from build123d import *

# Parameters (mm, degrees)
SKETCH1_R           = 16.5
BOSS_EXTRUDE1_DEPTH = 40
SKETCH2_R           = 1.25
CUT_EXTRUDE1_DEPTH  = 5
SKETCH3_R           = 5
BOSS_EXTRUDE2_DEPTH = 2.5
BOSS_EXTRUDE3_DEPTH = 8.5
CUT_EXTRUDE2_DEPTH  = 2
CUT_EXTRUDE3_START  = -16
SKETCH6_R           = 17.194108904
SKETCH6_R_2         = 15.5
CUT_EXTRUDE3_DEPTH  = 2
FILLET1_R           = 2
SKETCH7_R           = 4.1
BOSS_EXTRUDE4_DEPTH = 3
SKETCH8_R           = 2.5
BOSS_EXTRUDE5_DEPTH = 1
SKETCH9_W           = 3
SKETCH9_H           = 1
BOSS_EXTRUDE6_DEPTH = 6
CUT_EXTRUDE4_DEPTH  = 62.184148274
SKETCH11_W          = 1.5
SKETCH11_H          = 2.5
CUT_EXTRUDE5_DEPTH  = 62.184148274
CUT_EXTRUDE6_DEPTH  = 3.85
FILLET2_R           = 1


with BuildPart() as part:
    # Sketch1 → Boss-Extrude1 (new body)
    with BuildSketch(Plane.XY):
        Circle(SKETCH1_R)
    extrude(amount=BOSS_EXTRUDE1_DEPTH)

    # Sketch2 → Cut-Extrude1 (cut)
    with BuildSketch(Plane.XY.offset(40)):
        with Locations((0, 14)):
            Circle(SKETCH2_R)
        with Locations((12.124355653, -7)):
            Circle(SKETCH2_R)
        with Locations((-12.124355653, -7)):
            Circle(SKETCH2_R)
    extrude(amount=-CUT_EXTRUDE1_DEPTH, mode=Mode.SUBTRACT)

    # Sketch3 → Boss-Extrude2 (add)
    with BuildSketch(Plane.XY.offset(40)):
        with Locations((0, -7)):
            Circle(SKETCH3_R)
    extrude(amount=BOSS_EXTRUDE2_DEPTH)

    # Sketch4 → Boss-Extrude3 (add)
    with BuildSketch(Plane.XY.offset(42.5)):
        with BuildLine():
            Line((-2, -8.5), (2, -8.5))
            ThreePointArc((2, -8.5), (0, -4.5), (-2, -8.5))
        make_face()
    extrude(amount=BOSS_EXTRUDE3_DEPTH)

    # Sketch5 → Cut-Extrude2 (cut)
    with BuildSketch(Plane.XY.offset(40)):
        with BuildLine():
            Line((-13.5, 2.25), (-17.622574656, 2.25))
            Line((-17.622574656, 2.25), (-17.622574656, -2.25))
            Line((-17.622574656, -2.25), (-13.5, -2.25))
            ThreePointArc((-13.5, -2.25), (-11.25, 0), (-13.5, 2.25))
        make_face()
        with BuildLine():
            Line((17.622574656, -2.25), (13.5, -2.25))
            ThreePointArc((13.5, -2.25), (11.25, 0), (13.5, 2.25))
            Line((13.5, 2.25), (17.622574656, 2.25))
            Line((17.622574656, 2.25), (17.622574656, -2.25))
        make_face()
    extrude(amount=-CUT_EXTRUDE2_DEPTH, mode=Mode.SUBTRACT)

    # Sketch6 → Cut-Extrude3 (cut)
    with BuildSketch(Plane.XY.offset(40).offset(CUT_EXTRUDE3_START)):
        Circle(SKETCH6_R)
        Circle(SKETCH6_R_2, mode=Mode.SUBTRACT)
    extrude(amount=-CUT_EXTRUDE3_DEPTH, mode=Mode.SUBTRACT)

    # Fillet1
    # the kernel refuses this fillet: 2 mm, written as the material it takes off along each edge
    with BuildSketch(Plane(origin=(0, 0, 22), x_dir=(1, 0, 0), z_dir=(0, 1, 0))) as fillet1_piece_1:
        with BuildLine():
            CenterArc((14.5, 1.732050808), FILLET1_R, 300, 60)
            Line((15.5, 0), (15.52, -0.034641016))
            ThreePointArc((15.52, -0.034641016), (16, -0.04), (16.5, -0.04))
            Line((16.5, -0.04), (16.54, 0))
            Line((16.54, 0), (16.54, 1.732050808))
            Line((16.54, 1.732050808), (16.5, 1.732050808))
        make_face()
    revolve(axis=Axis((0, 0, 22), (0, 0, -1)), mode=Mode.SUBTRACT)

    # Sketch7 → Boss-Extrude4 (add)
    with BuildSketch(Plane(origin=(0, 0, 0), x_dir=(-1, 0, 0), z_dir=(0, 0, -1))):
        Circle(SKETCH7_R)
    extrude(amount=BOSS_EXTRUDE4_DEPTH)

    # Sketch8 → Boss-Extrude5 (add)
    with BuildSketch(Plane(origin=(0, 0, 0), x_dir=(-1, 0, 0), z_dir=(0, 0, -1))):
        with Locations(Location((0, 12.5, 0), (0, 0, 180))):
            Circle(SKETCH8_R)
        with Locations(Location((0, -12.5, 0), (0, 0, 180))):
            Circle(SKETCH8_R)
    extrude(amount=BOSS_EXTRUDE5_DEPTH)

    # Sketch9 → Boss-Extrude6 (add)
    with BuildSketch(Plane(origin=(0, 0, -1), x_dir=(-1, 0, 0), z_dir=(0, 0, -1))):
        with Locations((0, -12.5)):
            Rectangle(SKETCH9_W, SKETCH9_H)
        with Locations((0, 12.5)):
            Rectangle(SKETCH9_W, SKETCH9_H)
    extrude(amount=BOSS_EXTRUDE6_DEPTH)

    # Sketch10 → Cut-Extrude4 (cut, through all)
    with BuildSketch(Plane(origin=(0, 13, 0), x_dir=(1, 0, 0), z_dir=(0, 1, 0))):
        Polygon((-1.5, 7), (-0.5, 7), (-1.5, 6), align=None)
        Polygon((1.5, 7), (0.5, 7), (1.5, 6), align=None)
    extrude(amount=-CUT_EXTRUDE4_DEPTH, mode=Mode.SUBTRACT)

    # Sketch11 → Cut-Extrude5 (cut, through all)
    with BuildSketch(Plane(origin=(0, 13, 0), x_dir=(1, 0, 0), z_dir=(0, 1, 0))):
        with Locations((0, 4.75)):
            Rectangle(SKETCH11_W, SKETCH11_H)
    extrude(amount=-CUT_EXTRUDE5_DEPTH, mode=Mode.SUBTRACT)

    # Sketch12 → Cut-Extrude6 (cut)
    with BuildSketch(Plane(origin=(0, 0, 0), x_dir=(-1, 0, 0), z_dir=(0, 0, -1))):
        Polygon((7.778174593, 10.606601718), (11.692726543, 14.521153668), (14.527839542, 11.699412418), (10.606601718, 7.778174593), align=None)
        Polygon((10.606601718, -7.778174593), (14.521153668, -11.692726543), (11.699412418, -14.527839542), (7.778174593, -10.606601718), align=None)
        Polygon((-7.778174593, -10.606601718), (-11.692726543, -14.521153668), (-14.527839542, -11.699412418), (-10.606601718, -7.778174593), align=None)
        Polygon((-10.606601718, 7.778174593), (-14.521153668, 11.692726543), (-11.699412418, 14.527839542), (-7.778174593, 10.606601718), align=None)
    extrude(amount=-CUT_EXTRUDE6_DEPTH, mode=Mode.SUBTRACT)

    # Fillet2
    fillet2_edges = [part.edges().sort_by_distance(p)[0] for p in [
        (-11.66726189, 11.66726189, 3.85),
        (-11.66726189, -11.66726189, 3.85),
        (11.66726189, -11.66726189, 3.85),
        (11.66726189, 11.66726189, 3.85),
    ]]
    fillet(fillet2_edges, radius=FILLET2_R)


solid = part.part
Read the model definition and answer for the solid it produces. Units are mm, in the model's axes. A direction names the side the tool comes from. Coordinates: 2 decimals unless noted, no trailing zeros. Loops run counter-clockwise (first coordinate to the right, second up) from the corner with the lowest first, then second, coordinate; pieces in that order, holes last. Notation, with made-up numbers: (-13, -33.75) -> (45, -33.75) arc R29 ccw to (45, 2.25) -> close; hole circle Ø10 at (0, 77.5). An arc over 180 degrees is marked (long way). Answer in a Markdown table with one row per item.
Item 1: For a pull along X with two mould halves and no side action, classify faces 1 (the flat face through (9.212, -9.173, 1.898)), 2 (the flat face through (8.99, 11.82, 1.85)), 3 (the flat face through (-12, -7, 35)), 4 (the flat face through (-15, -2.25, 39)) as released by +X, released by -X, zero draft, split by the parting line, or undercut.
Returned:
| item | result |
|---|---|
| face 1 | undercut |
| face 2 | released by +X |
| face 3 | undercut |
| face 4 | zero draft |
Item 2: For faces 5 (the flat face through (-9.173, -9.212, 1.898)), 6 (the flat face through (0, 0, -3)), 7 (the flat face through (0, -8.5, 47)), 8 (the flat face through (14, 0, 38)), determine the directions among +Z, -Z, +X, -X, +Y, -Y from which every point of the face is accessible in a straight line to the end or side of a thin tool.
Returned:
| item | result |
|---|---|
| face 5 | -Z |
| face 6 | -Z, +X, -X |
| face 7 | +Z, +X, -X, -Y |
| face 8 | +Z, +X |
Item 3: A cutting plane is placed at B-B on z = 37. Determine the outline of the cut face in (x, y).
Returned:
| item | result |
|---|---|
| outline | circle Ø33 at (0, 0); hole circle Ø2.5 at (-12.12, -7); hole circle Ø2.5 at (0, 14); hole circle Ø2.5 at (12.12, -7) |
Item 4: Straight lines are drawn through the part: line 1 along Z through (x, y) = (-3, -7); line 2 along Z through (x, y) = (12, 9.5); line 3 along Y through (x, z) = (0, 36). For each, find the intervals that lie inside material, in ascending order. Write a range as [from, to].
Returned:
| item | result |
|---|---|
| line 1 | z = [0, 42.5] |
| line 2 | z = [3.85, 40] |
| line 3 | y = [-16.5, 12.75], [15.25, 16.5] |
Item 5: A cutting plane is placed at C-C on z = 23. Determine the outline of the cut face in (x, y), plus the area to 3 significant figures.
Returned:
| item | result |
|---|---|
| outline | circle Ø31 at (0, 0) |
| area | 755 mm^2 |
Item 6: A cutting plane is placed at A-A on y = 0. Determine the outline of the cut face in (x, z).
Returned:
| item | result |
|---|---|
| outline | (-16.5, 0) -> (-4.1, 0) -> (-4.1, -3) -> (4.1, -3) -> (4.1, 0) -> (16.5, 0) -> (16.5, 20.27) arc R2 ccw to (15.5, 22) -> (15.5, 24) -> (16.5, 24) -> (16.5, 38) -> (11.25, 38) -> (11.25, 40) -> (-11.25, 40) -> (-11.25, 38) -> (-16.5, 38) -> (-16.5, 24) -> (-15.5, 24) -> (-15.5, 22) arc R2 ccw to (-16.5, 20.27) -> close |
Item 7: Each of these flat-tipped pins is pushed along its axis until it touches: P1, Ø0.5, axis at y = 12.5, z = -5.5, coming from the -X side; P2, Ø10, axis at y = -11.5, z = 25, coming from the -X side; P3, Ø12, axis at x = 3, z = 6, coming from the -Y side; P4, Ø6, axis at x = 4.5, y = 7.5, coming from the +Z side. Where does it stop, or does it pass through?
Returned:
| item | result |
|---|---|
| P1 | stops at x = -1.5 |
| P2 | stops at x = -15.17 |
| P3 | stops at y = -16.5 |
| P4 | stops at z = 40 |
Item 8: A cutting plane is placed at D-D on z = 13. Determine the outline of the cut face in (x, y), plus the area to 3 significant figures.
Returned:
| item | result |
|---|---|
| outline | circle Ø33 at (0, 0) |
| area | 855 mm^2 |
